Design review of the part built by this model. Coordinates are the model's own, in mm. A direction names the side the tool comes from. Coordinates: 2 decimals unless noted, no trailing zeros. Order: outer loops, then holes, each group sorted by start corner. A loop starts at its lowest first (then second) coordinate and runs counter-clockwise, first axis right, second up. Notation, with made-up numbers: M -39.5,4.5 L -8.5,4.5 A10 ccw -8.5,19.5 Z; hole C -4.75,-7 d4. An arc over 180 degrees is marked long. Answer as a JSON object with one key per item and string values.
from build123d import *

# Parameters (mm, degrees)
SKETCH_1_R               = 4.25
EXTRUDE_1_DEPTH          = 5
EXTRUDE_2_DEPTH          = 5
PATTERN_CIRCULAR_1_COUNT = 11


with BuildPart() as part:
    # 草图1 → 凸台-拉伸1 (new body)
    with BuildSketch(Plane.XY):
        Circle(SKETCH_1_R)
        with BuildLine():
            Line((-1, 1.118033989), (-1, -1.118033989))
            ThreePointArc((-1, -1.118033989), (1.5, 0), (-1, 1.118033989))
        make_face(mode=Mode.SUBTRACT)
    extrude(amount=EXTRUDE_1_DEPTH)

    # 草图2 → 凸台-拉伸2 (add)
    with BuildSketch(Plane.XY):
        with BuildLine():
            ThreePointArc((6.364840058, 1.318639842), (6.41933804, 1.020832567), (6.459909598, 0.720810648))
            add(Edge.make_bspline(
                [(6.459909598, 0.720810648), (6.30503635, 0.573432081), (6.060220687, 0.372889718), (5.705124958, 0.167850699), (5.152234448, -0.07959703), (4.606066867, 0.004749759), (4.245132436, -0.203348467)],
                knots=[0, 0, 0, 0, 0.262447939, 0.385242457, 0.502396504, 1, 1, 1, 1], degree=3))
            ThreePointArc((4.245132436, -0.203348467), (4.197259488, 0.667467448), (3.972639872, 1.510176297))
            add(Edge.make_bspline(
                [(6.364840058, 1.318639842), (6.171889239, 1.410705831), (5.87694123, 1.5254125), (5.475758403, 1.610184636), (4.873382667, 1.67391663), (4.380322357, 1.424307057), (3.972639872, 1.510176297)],
                knots=[0, 0, 0, 0, 0.262447939, 0.385242457, 0.502396504, 1, 1, 1, 1], degree=3))
        make_face()
    extrude_2 = extrude(amount=EXTRUDE_2_DEPTH)

    # 阵列(圆周)1: 凸台-拉伸2 ×11 about axis
    pattern_circular_1_axis = Axis((0, 0, 5), (0, 0, -1))
    for i in range(1, PATTERN_CIRCULAR_1_COUNT):
        add(extrude_2.rotate(pattern_circular_1_axis, i * 360 / PATTERN_CIRCULAR_1_COUNT))


solid = part.part
1) Tool access review of faces 1 (the flat face through (2, 0, 5)), 2 (the flat face through (-1, 0, 2)): name each direction out of +Z, -Z, +X, -X, +Y, -Y from which nothing blocks a thin tool from reaching the whole face with its end or side.
Taken from the geometry:
{"face 1": "+Z, +X, -X, +Y, -Y", "face 2": "+Z, -Z"}
2) To check wall thickness, follow L1, parallel to Y at x = -5, z = 4; L2, parallel to X at y = 3.75, z = 0.95; L3, parallel to Y at x = 0, z = 1.6. State the ranges of each line that lie inside material, in increasing order.
Taken from the geometry:
{"L1": "y = -3.1 to -1.48, -0.17 to 1.46, 3.47 to 4.15", "L2": "x = -5.11 to -3.21, -2.06 to 2, 3 to 4.94", "L3": "y = -6.5 to -1.5, 1.5 to 4.25"}
3) Add section A-A (x = 0). State the section outline as (y, z) points.
Taken from the geometry:
{"outline": "M -6.5,0 L -1.5,0 L -1.5,5 L -6.5,5 Z; M 1.5,0 L 4.25,0 L 4.25,5 L 1.5,5 Z"}
4) Insertion check: pin 1 Ø1.5 at (x, z) = (2, 2.5) entering from -Y. The pin has a flat end and moves straight along its axis. Give the tip position at first contact, or say it passes through.
Taken from the geometry:
{"pin 1": "stops at y = -5.28"}
5) Mouldability with a two-part tool opening along Y and no side actions: class faces 3 (the cylindrical face through (1.5, 0, 2.5)), 4 (the flat face through (2, 0, 0)) as released by +Y, released by -Y, zero draft, split by the parting line, or undercut.
Taken from the geometry:
{"face 3": "undercut", "face 4": "zero draft"}
